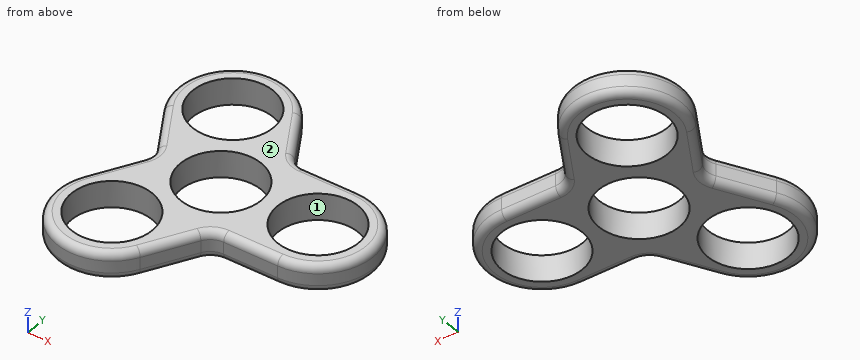
from build123d import *

# Parameters (mm, degrees)
F0_R     = 11
F1_DEPTH = 7.25
F2_R     = 5
F3_R     = 2


with BuildPart() as f1:
    # F0 (on Top) → F1 (new body)
    with BuildSketch(Plane.XY):
        with BuildLine():
            Line((8.6602539087, -14.9999997764), (25.9999998066, -15))
            ThreePointArc((25.9999998066, -15), (41, 0), (25.9999998066, 15))
            Line((25.9999998066, 15), (8.6602539087, 14.9999997764))
            Line((8.6602539087, 14.9999997764), (-0.0096188465, 30.0166603309))
            ThreePointArc((-0.0096188465, 30.0166603309), (-20.5, 35.5070415552), (-25.9903809601, 15.0166603309))
            Line((-25.9903809601, 15.0166603309), (-17.3205078175, 0))
            Line((-17.3205078175, 0), (-25.9903809601, -15.0166603309))
            ThreePointArc((-25.9903809601, -15.0166603309), (-20.5, -35.5070415552), (-0.0096188465, -30.0166603309))
            Line((-0.0096188465, -30.0166603309), (8.6602539087, -14.9999997764))
        make_face()
        with Locations((-13, -22.5166604984)):
            Circle(F0_R, mode=Mode.SUBTRACT)
        Circle(F0_R, mode=Mode.SUBTRACT)
        with BuildLine():
            ThreePointArc((37, 0), (26, -11), (15, 0))
            ThreePointArc((15, 0), (26, 11), (37, 0))
        make_face(mode=Mode.SUBTRACT)
        with Locations((-13, 22.5166604984)):
            Circle(F0_R, mode=Mode.SUBTRACT)
    extrude(amount=F1_DEPTH)

    # F2
    f2_edges = [f1.edges().sort_by_distance(p)[0] for p in [
        (8.660254, 15, 3.625),
        (-17.320508, 0, 3.625),
        (8.660254, -15, 3.625),
    ]]
    fillet(f2_edges, radius=F2_R)

    # F3
    f3_edges = [f1.edges().sort_by_distance(p)[0] for p in [
        (3.60363, -23.75833, 7.25),
        (-20.5, -35.507042, 7.25),
        (-22.377132, -8.75833, 7.25),
        (-18.094011, 0, 7.25),
        (-22.377132, 8.75833, 7.25),
        (-20.5, 35.507042, 7.25),
        (3.60363, 23.75833, 7.25),
        (18.773503, 15, 7.25),
        (41, 0, 7.25),
        (18.773503, -15, 7.25),
        (9.047005, -15.669873, 7.25),
        (9.047005, 15.669873, 7.25),
        (18.773503, -15, 0),
        (3.60363, -23.75833, 0),
        (-22.377132, -8.75833, 0),
        (-20.5, -35.507042, 0),
        (41, 0, 0),
        (18.773503, 15, 0),
        (-20.5, 35.507042, 0),
        (3.60363, 23.75833, 0),
        (-22.377132, 8.75833, 0),
        (-18.094011, 0, 0),
        (9.047005, 15.669873, 0),
        (9.047005, -15.669873, 0),
    ]]
    fillet(f3_edges, radius=F3_R)


solid = f1.part
Geometry check sheet. Reference: the model listing, model coordinates, mm. Face numbers are marked on the shaded views. Give positions to 0.01 mm unless a question says otherwise; leave off trailing zeros. Loops run counter-clockwise (first coordinate to the right, second up) from the corner with the lowest first, then second, coordinate; pieces in that order, holes last. Notation, with made-up numbers: (87.25, 58.5) -> (132.25, 58.5) arc R20 ccw to (132.25, 88.5) -> close; hole circle Ø8 at (-9.75, 75.5). An arc over 180 degrees is marked (long way). Answer in a Markdown table with one row per item. Add a question column.
1) Cross-section at B-B on x = -13. State how many separate pieces and enclosed holes the cut face has, and give its area (3 significant figures).
2) Material ranges on probe 1 along Y at (x, z) = (-20, 5); probe 2 along X at (y, z) = (-4, 1); probe 3 along X at (y, z) = (-8, 0.75), recorded low to high. Write a range as from..to.
3) Draft check along Y on the marked faces 1 and 2. Enter one of: pulls with the +Y half, pulls with the -Y half, needs draft (parallel to the pull), parting line crosses it, or undercut.
4) Cross-section at A-A on y = 0. Record the boundary of the cut face in (x, z), and give its area (3 significant figures).
5) Gauge pin test, flat ends, axial feed: P1, Ø3, axis at y = 1.5, z = 2, coming from the +X side; P2, Ø17.5, axis at x = 26, y = 0, coming from the +Z side; P3, Ø1.6, axis at x = 20, z = 4.5, coming from the -Y side; P4, Ø3, axis at y = 13, z = 4, coming from the +X side. Record the tip position at first contact, or that the pin passes through.
Outcome:
| question | item | result |
|---|---|---|
| 1 | separate pieces | 3 |
| 1 | enclosed holes | 0 |
| 1 | area | 222 mm^2 |
| 2 | probe 1 | y = -35.78..-31, -14.03..-4.64, 4.64..14.03, 31..35.78 |
| 2 | probe 2 | x = -19.32..-10.25, 10.25..15.75, 36.25..40.18 |
| 2 | probe 3 | x = -21.43..-7.55, 7.55..18.45, 33.55..38.17 |
| 3 | face 1 | undercut |
| 3 | face 2 | needs draft |
| 4 | outline | (-18.09, 2) arc R2 ccw to (-16.09, 0) -> (-11, 0) -> (-11, 7.25) -> (-16.09, 7.25) arc R2 ccw to (-18.09, 5.25) -> close; (11, 0) -> (15, 0) -> (15, 7.25) -> (11, 7.25) -> close; (37, 0) -> (39, 0) arc R2 ccw to (41, 2) -> (41, 5.25) arc R2 ccw to (39, 7.25) -> (37, 7.25) -> close |
| 4 | area | 106 mm^2 |
| 5 | P1 | stops at x = 41 |
| 5 | P2 | passes through |
| 5 | P3 | stops at y = -15 |
| 5 | P4 | stops at x = 35.63 |
